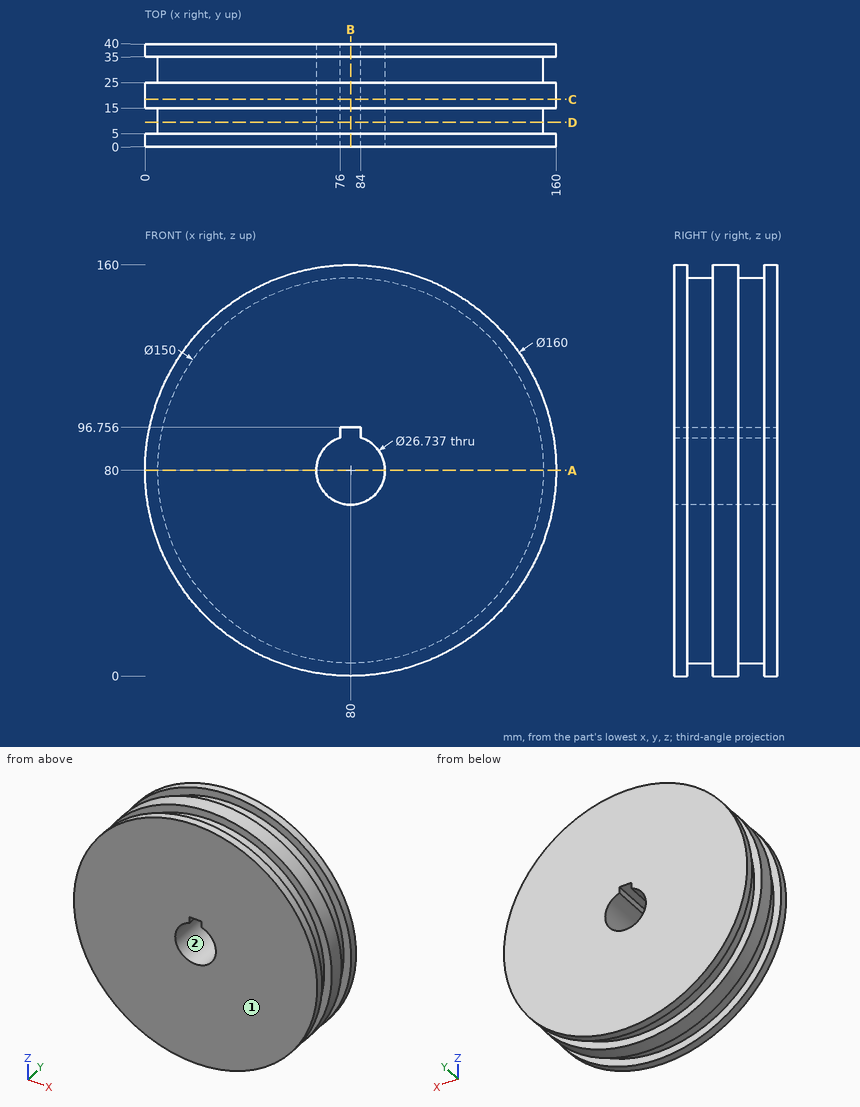
Answer from the drawing. Dimensions are ordinates in mm from the lowest x, y and z of the part. Round coordinates to 2 decimals unless told otherwise and drop trailing zeros. Order: outer loops, then holes, each group sorted by start corner. A loop starts at its lowest first (then second) coordinate and runs counter-clockwise, first axis right, second up.
1) The mould has two halves that part along X. Classify the marked faces 1 and 2: released by +X, released by -X, zero draft, split by the parting line, or undercut.
2) The part is cut by section C-C on y = 18.5. Write down the section's boundary in (x, z), plus the area to 3 significant figures.
3) Flat-ended cylindrical pins translate along their axes: pin 1 (3 mm diameter, centred on y = 14.5, z = 50.5, fed in from +X); pin 2 (24 mm diameter, centred on x = 80, z = 80, fed in from +Y); pin 3 (2 mm diameter, centred on y = 13.5, z = 24, fed in from +X); pin 4 (4 mm diameter, centred on y = 34.5, z = 83.5, fed in from -X). Find the tip coordinate at first contact, or state that the pin passes through.
4) The part is cut by section D-D on y = 9.5. Write down the section's boundary in (x, z).
5) The part is cut by section A-A on z = 80. Write down the section's boundary in (x, y), plus the area to 3 significant figures.
6) Straight lines are drawn through the part: L1, parallel to Z at x = 80, y = 13; L2, parallel to X at y = 24.5, z = 80; L3, parallel to Z at x = 80, y = 19. For each, find the intervals that lie inside material, in ascending order.
7) The part is cut by section B-B on x = 80. Write down the section's boundary in (y, z), plus the area to 4 significant figures.
Resolved:
1. face 1: zero draft
1. face 2: undercut
2. outline: circle Ø160 at (80, 80); hole (76, 92.76) arc R13.37 ccw (long way) to (84, 92.76) - (84, 96.76) - (76, 96.76) - close
2. area: 19,500 mm2
3. pin 1: stops at x = 154.91
3. pin 2: passes through
3. pin 3: stops at x = 130.99
3. pin 4: stops at x = 0.02
4. outline: circle Ø150 at (80, 80); hole (76, 92.76) arc R13.37 ccw (long way) to (84, 92.76) - (84, 96.76) - (76, 96.76) - close
5. outline: (0, 0) - (66.63, 0) - (66.63, 40) - (0, 40) - (0, 35) - (5, 35) - (5, 25) - (0, 25) - (0, 15) - (5, 15) - (5, 5) - (0, 5) - close; (93.37, 0) - (160, 0) - (160, 5) - (155, 5) - (155, 15) - (160, 15) - (160, 25) - (155, 25) - (155, 35) - (160, 35) - (160, 40) - (93.37, 40) - close
5. area: 5,130 mm2
6. L1: z = 5 to 66.63, 96.76 to 155
6. L2: x = 0 to 66.63, 93.37 to 160
6. L3: z = 0 to 66.63, 96.76 to 160
7. outline: (0, 0) - (5, 0) - (5, 5) - (15, 5) - (15, 0) - (25, 0) - (25, 5) - (35, 5) - (35, 0) - (40, 0) - (40, 66.63) - (0, 66.63) - close; (0, 96.76) - (40, 96.76) - (40, 160) - (35, 160) - (35, 155) - (25, 155) - (25, 160) - (15, 160) - (15, 155) - (5, 155) - (5, 160) - (0, 160) - close
7. area: 4,995 mm2
